from build123d import *

# Parameters (mm, degrees)
SKETCH_R     = 3.5
PAD_DEPTH    = 2
SKETCH001_R  = 2
PAD001_DEPTH = 9.5
SKETCH002_R  = 1.5
PAD002_DEPTH = 3
SKETCH003_R  = 2
PAD003_DEPTH = 1


with BuildPart() as part:
    # Sketch → Pad (new body)
    with BuildSketch(Plane.XY):
        Circle(SKETCH_R)
    extrude(amount=PAD_DEPTH)

    # Sketch001 (on Face3 of Pad) → Pad001 (join)
    with BuildSketch(Plane.XY.offset(2)):
        Circle(SKETCH001_R)
    extrude(amount=PAD001_DEPTH)

    # Sketch002 (on Face5 of Pad001) → Pad002 (join)
    with BuildSketch(Plane.XY.offset(11.5)):
        Circle(SKETCH002_R)
    extrude(amount=PAD002_DEPTH)

    # Sketch003 (on Face7 of Pad002) → Pad003 (join)
    with BuildSketch(Plane.XY.offset(14.5)):
        Circle(SKETCH003_R)
    extrude(amount=PAD003_DEPTH)


solid = part.part
Work out the finished part from the listing and answer in its coordinate system (mm). A direction names the side the tool comes from. Coordinates: 2 decimals unless noted, no trailing zeros. Write each loop counter-clockwise with the first axis right and the second up, starting at its lowest first coordinate (ties: lowest second). Pieces come first, ordered by that corner, then holes. Notation, with made-up numbers: M -8.5,81.25 L 43.5,81.25 A16 cw 43.5,97.25 Z; hole C -26,4.5 d7. An arc over 180 degrees is marked long. Use one line per item in the form item = value. Start each with the question number.
1. The part is cut by section A-A (y = 0). Give the vertices of the cut face in (x, z).
2. A tool of negligible diameter and unlimited length cuts with its end or side. For faces 1 (the face through (0, -2, 7)), 2 (the face through (0, 0, 15.5)), from which of +Z, -Z, +X, -X, +Y, -Y can it reach the whole face along a straight path? Write none if from no direction.
3. The mould has two halves that part along Z. Classify faces 3 (the face through (-1.5, 0.07, 12.98)), 4 (the face through (0, -2, 15)), 5 (the face through (2, -2, 2)): released by +Z, released by -Z, zero draft, split by the parting line, or undercut.
4. Straight lines are drawn through the part: probe 1 along Z at (x, y) = (-1, -1.25); probe 2 along Z at (x, y) = (-1.5, -2); probe 3 along X at (y, z) = (-1.5, 9.75). For each, find the intervals that lie inside material, in ascending order. Write a range as from..to.
5. The part is cut by section C-C (z = 10.75). Give the vertices of the cut face in (x, y), plus the area to 3 significant figures.
6. The part is cut by section D-D (y = 2.25). Give the vertices of the cut face in (x, z), plus the area to 3 significant figures.
7. Each of these flat-tipped pins is pushed along its axis until it touches: P1, Ø1, axis at y = 0.5, z = 9.5, coming from the +X side; P2, Ø2, axis at x = 1.5, z = 11.5, coming from the -Y side; P3, Ø1, axis at y = -1.5, z = 9.5, coming from the -X side. Where does it stop, or does it pass through?
Evaluation:
q1.outline = M -3.5,0 L 3.5,0 L 3.5,2 L 2,2 L 2,11.5 L 1.5,11.5 L 1.5,14.5 L 2,14.5 L 2,15.5 L -2,15.5 L -2,14.5 L -1.5,14.5 L -1.5,11.5 L -2,11.5 L -2,2 L -3.5,2 Z
q2.face_1 = +Z
q2.face_2 = +Z, +X, -X, +Y, -Y
q3.face_3 = undercut
q3.face_4 = zero draft
q3.face_5 = released by +Z
q4.probe_1 = 0..11.5, 14.5..15.5
q4.probe_2 = 0..2
q4.probe_3 = -1.32..1.32
q5.outline = C 0,0 d4
q5.area = 12.6 mm^2
q6.outline = M -2.68,0 L 2.68,0 L 2.68,2 L -2.68,2 Z
q6.area = 10.7 mm^2
q7.P1 = 2
q7.P2 = -1.94
q7.P3 = -1.73
